```python
from build123d import *

# Parameters (mm, degrees)
ESQUISSE1_W             = 17
ESQUISSE1_H             = 11
ESQUISSE1_R             = 1.75
BOSS_EXTRU_1_DEPTH      = 5
ESQUISSE2_W             = 2
ESQUISSE2_H             = 7
BOSS_EXTRU_2_DEPTH      = 20
ESQUISSE3_W             = 4
ESQUISSE3_H             = 7
ENL_V_MAT_EXTRU_1_DEPTH = 20
ESQUISSE4_R             = 1.25
ESQUISSE4_W             = 5
ESQUISSE4_H             = 20
ENL_V_MAT_EXTRU_2_DEPTH = 20
ESQUISSE5_R             = 2.95
ENL_V_MAT_EXTRU_3_DEPTH = 2.5
CONG_1_START            = -11
CONG_1_DEPTH            = 11
CONG_1_2_DEPTH          = 2
CONG_1_START_2          = -2
CONG_1_3_DEPTH          = 2


with BuildPart() as part:
    # Esquisse1 → Boss.-Extru.1 (new body)
    with BuildSketch(Plane.XY):
        with Locations((8.5, -5.5)):
            Rectangle(ESQUISSE1_W, ESQUISSE1_H)
        with Locations((5.5, -5.5)):
            Circle(ESQUISSE1_R, mode=Mode.SUBTRACT)
        with Locations((11.5, -5.5)):
            Circle(ESQUISSE1_R, mode=Mode.SUBTRACT)
    extrude(amount=BOSS_EXTRU_1_DEPTH)

    # Esquisse2 → Boss.-Extru.2 (add)
    with BuildSketch(Plane.XY.offset(5)):
        Polygon((15, -9), (0, -9), (0, -11), (17, -11), (17, -9), align=None)
        with Locations((16, -5.5)):
            Rectangle(ESQUISSE2_W, ESQUISSE2_H)
        Polygon((17, 0), (0, 0), (0, -2), (15, -2), (17, -2), align=None)
    extrude(amount=BOSS_EXTRU_2_DEPTH)

    # Esquisse3 → Enlèv. mat.-Extru.1 (cut)
    with BuildSketch(Plane.ZY.offset(-15)):
        with Locations((7, -5.5)):
            Rectangle(ESQUISSE3_W, ESQUISSE3_H)
        with Locations((23, -5.5)):
            Rectangle(ESQUISSE3_W, ESQUISSE3_H)
        with Locations((16, -5.5)):
            Rectangle(ESQUISSE3_W, ESQUISSE3_H)
    extrude(amount=-ENL_V_MAT_EXTRU_1_DEPTH, mode=Mode.SUBTRACT)

    # Esquisse4 → Enlèv. mat.-Extru.2 (cut)
    with BuildSketch(Plane(origin=(0, -11, 0), x_dir=(-1, 0, 0), z_dir=(0, -1, 0))):
        with Locations(Location((-11.5, -20, 0), (0, 0, 90))):
            Circle(ESQUISSE4_R)
        with Locations(Location((-11.5, -10.5, 0), (0, 0, 90))):
            Circle(ESQUISSE4_R)
        with Locations((-2.5, -15)):
            Rectangle(ESQUISSE4_W, ESQUISSE4_H)
    extrude(amount=-ENL_V_MAT_EXTRU_2_DEPTH, mode=Mode.SUBTRACT)

    # Esquisse5 → Enlèv. mat.-Extru.3 (cut)
    with BuildSketch(Plane.XY.offset(5)):
        with Locations((5.5, -5.5)):
            Circle(ESQUISSE5_R)
        with Locations((11.5, -5.5)):
            Circle(ESQUISSE5_R)
    extrude(amount=-ENL_V_MAT_EXTRU_3_DEPTH, mode=Mode.SUBTRACT)

    # Congé1: read off the stored shape, not the designer's step
    # Congé1 outline → Congé1 (cut)
    with BuildSketch(Plane(origin=(0, 0, 0), x_dir=(1, 0, 0), z_dir=(0, 1, 0)).offset(CONG_1_START)):
        with BuildLine():
            ThreePointArc((8, -25), (5.878679656, -24.121320344), (5, -22))
            Line((5, -22), (5, -25))
            Line((5, -25), (8, -25))
        make_face()
    extrude(amount=CONG_1_DEPTH, mode=Mode.SUBTRACT)

    # Cong_1 2 outline → Cong_1 2 (add)
    with BuildSketch(Plane(origin=(0, 0, 0), x_dir=(1, 0, 0), z_dir=(0, 1, 0)).offset(CONG_1_START)):
        with BuildLine():
            ThreePointArc((2, -5), (4.121320344, -5.878679656), (5, -8))
            Line((5, -8), (5, -5))
            Line((5, -5), (2, -5))
        make_face()
    extrude(amount=CONG_1_2_DEPTH)

    # Cong_1 3 outline → Cong_1 3 (add)
    with BuildSketch(Plane(origin=(0, 0, 0), x_dir=(1, 0, 0), z_dir=(0, 1, 0)).offset(CONG_1_START_2)):
        with BuildLine():
            ThreePointArc((2, -5), (4.121320344, -5.878679656), (5, -8))
            Line((5, -8), (5, -5))
            Line((5, -5), (2, -5))
        make_face()
    extrude(amount=CONG_1_3_DEPTH)


solid = part.part
```
Design review of the part built by this model. Coordinates are the model's own, in mm. A direction names the side the tool comes from. Coordinates: 2 decimals unless noted, no trailing zeros. Order: outer loops, then holes, each group sorted by start corner. A loop starts at its lowest first (then second) coordinate and runs counter-clockwise, first axis right, second up. Notation, with made-up numbers: M 42,-18 L 50,-18 A19 ccw 50,5 Z; hole C 51.25,86.5 d8. An arc over 180 degrees is marked long. Answer as a JSON object with one key per item and string values. Group by question number.
1) Add section A-A, the plane x = 11.5. Count the separate pieces of the cut face and the enclosed holes in it, then the cut area to 3 significant figures.
2) Add section D-D, the plane x = 5.5. Write out the cut boundary in (y, z).
3) Wall thickness on L1, parallel to X at y = -5.5, z = 1.85; L2, parallel to X at y = -1.1, z = 20; L3, parallel to Y at x = 16.25, z = 21.5: over which ranges is each line inside the solid? List them lowest first.
4) Add section B-B, the plane z = 20. Write out the cut boundary in (x, y).
5) Tool access review of faces 1 (the flat face through (8.5, -6.7, 5)), 2 (the flat face through (15, -6, 11)), 3 (the flat face through (16, -6, 21)): name each direction out of +Z, -Z, +X, -X, +Y, -Y from which nothing blocks a thin tool from reaching the whole face with its end or side.
6) Mouldability with a two-part tool opening along X and no side actions: class faces 4 (the flat face through (16, -6, 9)), 5 (the cylindrical face through (12.554, -10.014, 19.328)), 6 (the cylindrical face through (5.9, -10.01, 24.14)), 7 (the cylindrical face through (12.345, -1.014, 11.421)) as pulls with the +X half, pulls with the -X half, needs draft (parallel to the pull), parting line crosses it, or undercut.
7) Add section C-C, the plane y = -5.5. Write out the cut boundary in (x, z).
8) For pin 1 (2.5 mm diameter, centred on y = -7, z = 12.5, fed in from -X); pin 2 (1 mm diameter, centred on y = -3, z = 15, fed in from -X); pin 3 (2 mm diameter, centred on y = -10.5, z = 18.5, fed in from -X); pin 4 (4 mm diameter, centred on x = 11.5, y = -5.5, fed in from +Z), all flat-tipped, find the tip position at first contact; note any pin that passes through.
Computed values:
{
 "1": {"separate pieces": "6", "enclosed holes": "0", "area": "91.5 mm^2"},
 "2": {"outline": "M -11,0 L -7.25,0 L -7.25,2.5 L -8.45,2.5 L -8.45,5 L -9,5 L -9,23.66 L -11,23.66 Z; M -3.75,0 L 0,0 L 0,23.66 L -2,23.66 L -2,5 L -2.55,5 L -2.55,2.5 L -3.75,2.5 Z"},
 "3": {"L1": "x = 0 to 3.75, 7.25 to 9.75, 13.25 to 17", "L2": "x = 5 to 10.25, 12.75 to 17", "L3": "y = -11 to -9, -2 to 0"},
 "4": {"outline": "M 5,-11 L 10.25,-11 L 10.25,-9 L 5,-9 Z; M 5,-2 L 10.25,-2 L 10.25,0 L 5,0 Z; M 12.75,-11 L 17,-11 L 17,0 L 12.75,0 L 12.75,-2 L 15,-2 L 15,-9 L 12.75,-9 Z"},
 "5": {"face 1": "-X", "face 2": "+Z, -X", "face 3": "+Z, +X, -X"},
 "6": {"face 4": "needs draft", "face 5": "undercut", "face 6": "pulls with the -X half", "face 7": "undercut"},
 "7": {"outline": "M 0,0 L 3.75,0 L 3.75,2.5 L 2.55,2.5 L 2.55,5 L 0,5 Z; M 7.25,0 L 9.75,0 L 9.75,2.5 L 8.55,2.5 L 8.55,5 L 8.45,5 L 8.45,2.5 L 7.25,2.5 Z; M 13.25,0 L 17,0 L 17,5 L 14.45,5 L 14.45,2.5 L 13.25,2.5 Z; M 15,9 L 17,9 L 17,14 L 15,14 Z; M 15,18 L 17,18 L 17,21 L 15,21 Z"},
 "8": {"pin 1": "stops at x = 15", "pin 2": "passes through", "pin 3": "stops at x = 5", "pin 4": "stops at z = 2.5"}
}
